CAD build for the part. Positions are in the model's coordinates, mm. Face numbers are marked on the shaded views. Coordinates: 2 decimals unless noted, no trailing zeros. Write each loop counter-clockwise with the first axis right and the second up, starting at its lowest first coordinate (ties: lowest second). Pieces come first, ordered by that corner, then holes. Notation, with made-up numbers: (21, 49.5) -> (55, 49.5) arc R19 ccw to (55, 84.5) -> close; hole circle Ø7 at (5.5, 41.25). An arc over 180 degrees is marked (long way). Answer as CSV lines item,"result". Start each with the question number.
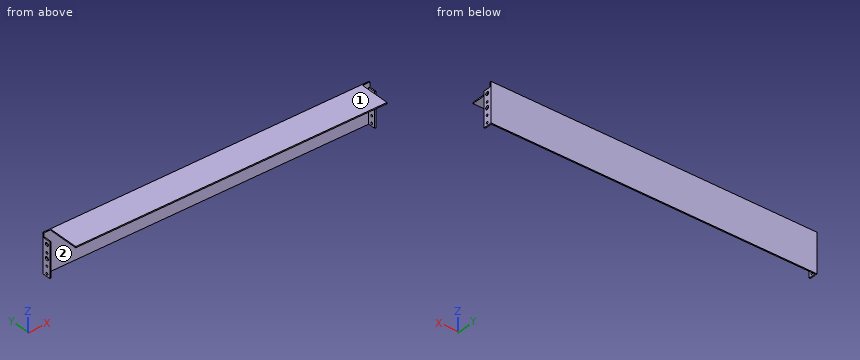
```python
from build123d import *

# Parameters (mm, degrees)
SKETCH1_W           = 700
SKETCH1_H           = 70
BOSS_EXTRUDE1_DEPTH = 2.6
SKETCH2_W           = 733
SKETCH2_H           = 88
BOSS_EXTRUDE2_DEPTH = 2.6
SKETCH3_W           = 77.5
SKETCH3_H           = 16.4
SKETCH3_R           = 2.5
SKETCH3_R_2         = 4
BOSS_EXTRUDE3_DEPTH = 2.6
BOSS_EXTRUDE4_START = -2.6
SKETCH4_W           = 77.5
SKETCH4_H           = 16.4
SKETCH4_R           = 2.5
SKETCH4_R_2         = 4
BOSS_EXTRUDE4_DEPTH = 2.6


with BuildPart() as part:
    # Sketch1 → Boss-Extrude1 (new body)
    with BuildSketch(Plane.XY):
        Rectangle(SKETCH1_W, SKETCH1_H)
    extrude(amount=-BOSS_EXTRUDE1_DEPTH)

    # Sketch2 → Boss-Extrude2 (add)
    with BuildSketch(Plane(origin=(0, 35, 0), x_dir=(1, 0, 0), z_dir=(0, 1, 0))):
        with Locations((0, 44)):
            Rectangle(SKETCH2_W, SKETCH2_H)
    extrude(amount=-BOSS_EXTRUDE2_DEPTH)

    # Sketch3 → Boss-Extrude3 (add)
    with BuildSketch(Plane.ZY.offset(366.5)):
        with Locations((-49.25, 24.2)):
            Rectangle(SKETCH3_W, SKETCH3_H)
        with Locations(Location((-82, 24.2, 0), (0, 0, 270))):
            Circle(SKETCH3_R, mode=Mode.SUBTRACT)
        with Locations(Location((-66, 24.2, 0), (0, 0, 270))):
            Circle(SKETCH3_R, mode=Mode.SUBTRACT)
        with Locations(Location((-50, 24.2, 0), (0, 0, 270))):
            Circle(SKETCH3_R_2, mode=Mode.SUBTRACT)
        with Locations(Location((-38, 24.2, 0), (0, 0, 270))):
            Circle(SKETCH3_R, mode=Mode.SUBTRACT)
        with Locations(Location((-20, 24.2, 0), (0, 0, 270))):
            Circle(SKETCH3_R_2, mode=Mode.SUBTRACT)
    extrude(amount=-BOSS_EXTRUDE3_DEPTH)

    # Sketch4 → Boss-Extrude4 (add)
    with BuildSketch(Plane(origin=(366.5, 0, 0), x_dir=(0, 0, -1), z_dir=(1, 0, 0)).offset(BOSS_EXTRUDE4_START)):
        with Locations((49.25, 24.2)):
            Rectangle(SKETCH4_W, SKETCH4_H)
        with Locations(Location((38, 24.2, 0), (0, 0, 270))):
            Circle(SKETCH4_R, mode=Mode.SUBTRACT)
        with Locations(Location((50, 24.2, 0), (0, 0, 270))):
            Circle(SKETCH4_R_2, mode=Mode.SUBTRACT)
        with Locations(Location((66, 24.2, 0), (0, 0, 270))):
            Circle(SKETCH4_R, mode=Mode.SUBTRACT)
        with Locations(Location((82, 24.2, 0), (0, 0, 270))):
            Circle(SKETCH4_R, mode=Mode.SUBTRACT)
        with Locations(Location((20, 24.2, 0), (0, 0, 270))):
            Circle(SKETCH4_R_2, mode=Mode.SUBTRACT)
    extrude(amount=BOSS_EXTRUDE4_DEPTH)


solid = part.part
```
1. Cut at B-B (y = -18.5). Give the cut face in (x, z).
2. Flat gauge pins, fed straight in: P1, Ø1.3, axis at y = -9.5, z = -1.5, coming from the -X side; P2, Ø6, axis at x = -171.5, y = 27, coming from the -Z side; P3, Ø8, axis at y = 24.2, z = -82, coming from the -X side; P4, Ø1.5, axis at x = -239, z = -28.5, coming from the -Y side. Where does each tip first touch, or does it go through?
3. Mould opens along X. For the marked faces 1 and 2 say: pulls with the +X half, pulls with the -X half, needs draft (parallel to the pull), parting line crosses it, or undercut.
4. Wall check: line 1 (Z direction, x = 364.5, y = 24.2); line 2 (X direction, y = 23, z = -77); line 3 (Y direction, x = 365.7, z = -20). Give the ranges that are in metal, low to high.
5. Cut at A-A (x = 271). Give the cut face in (y, z), then the cut area to 3 significant figures.
Geometry check:
1,outline,"(-350, -2.6) -> (350, -2.6) -> (350, 0) -> (-350, 0) -> close"
2,P1,"x = -350"
2,P2,"z = -2.6"
2,P3,"x = -366.5"
2,P4,"y = 32.4"
3,face 1,"needs draft"
3,face 2,"undercut"
4,line 1,"-88 to -84.5, -79.5 to -68.5, -63.5 to -54, -46 to -40.5, -35.5 to -24, -16 to -10.5"
4,line 2,"-366.5 to -363.9, 363.9 to 366.5"
4,line 3,"16 to 20.2, 28.2 to 35"
5,outline,"(-35, -2.6) -> (32.4, -2.6) -> (32.4, -88) -> (35, -88) -> (35, 0) -> (-35, 0) -> close"
5,area,"404 mm²"
